Check sheet for the drawn part. Datum: minimum x, y, z corner. Units: mm. A direction names the side the tool comes from. Coordinates: 2 decimals unless noted, no trailing zeros. Write each loop counter-clockwise with the first axis right and the second up, starting at its lowest first coordinate (ties: lowest second). Pieces come first, ordered by that corner, then holes. Notation, with made-up numbers: (57, 6) -> (78, 6) arc R14 cw to (78, 31) -> close; hole circle Ø9 at (-12.75, -29). An arc over 180 degrees is marked (long way). Write item = value, one per line. Start each with the question number.
(1) Section check B-B (y = 9). Record the cut outline in (x, z), plus the area to 3 significant figures.
(2) Section check D-D (y = 19). Record the cut outline in (x, z), plus the area to 3 significant figures.
(3) Section check C-C (x = 32.5). Record the cut outline in (y, z), plus the area to 3 significant figures.
(4) Material ranges on probe 1 along Y at (x, z) = (32.5, 1.65); probe 2 along Y at (x, z) = (10, 0.8); probe 3 along Y at (x, z) = (20.5, 6), recorded low to high. Write a range as [from, to].
(5) Set-up check for the marked faces 1, 2 and 3: record each of +Z, -Z, +X, -X, +Y, -Y from which the full face is reachable in a straight line by a thin tool's end or side.
(6) Section check A-A (y = 42.5). Record the cut outline in (x, z), plus the area to 3 significant figures.
(7) Gauge pin test, flat ends, axial feed: pin 1 Ø3 at (y, z) = (35.5, 3) entering from -X; pin 2 Ø10 at (y, z) = (10, 4) entering from +X; pin 3 Ø3 at (x, y) = (23.5, 14) entering from +Z. Record the tip position at first contact, or that the pin passes through.
(8) Mould release check, pull along Y, two halves, no side actions. Record for the marked faces 4, 5 and 6: released by +Y, released by -Y, zero draft, split by the parting line, or undercut.
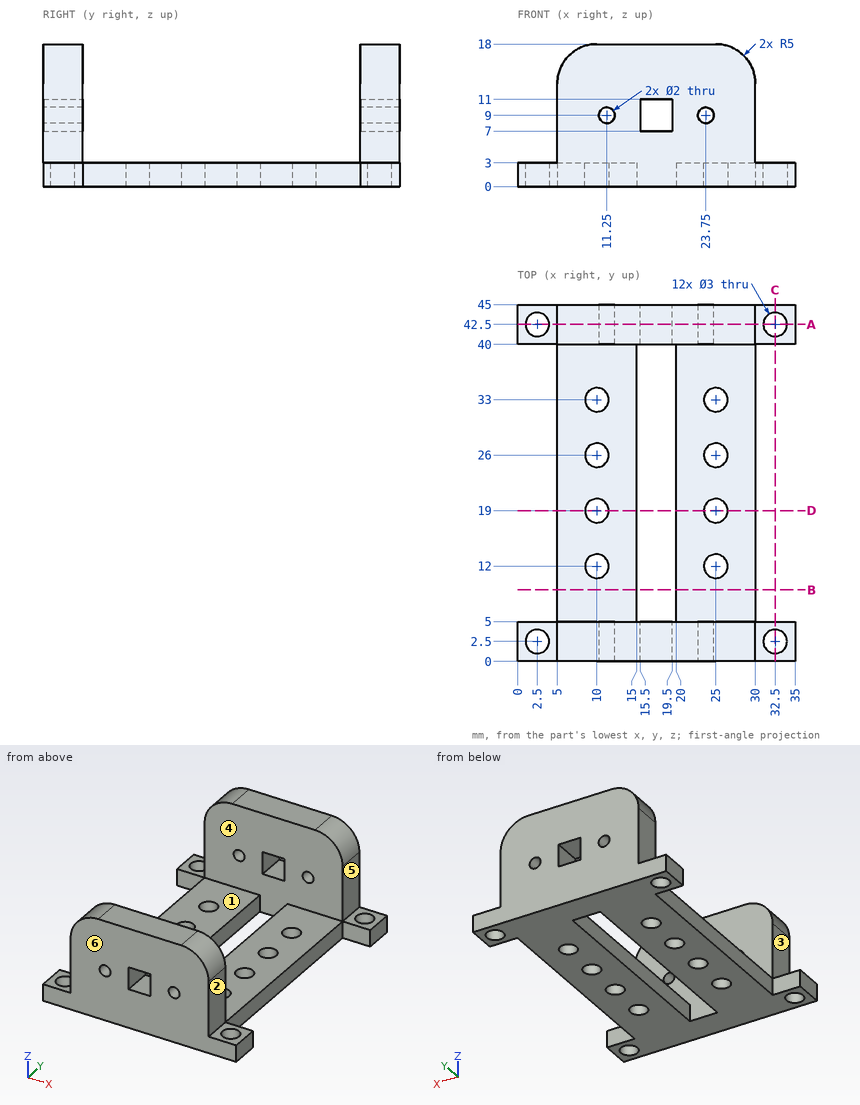
Response:
q1.outline = (5, 0) -> (15, 0) -> (15, 3) -> (5, 3) -> close; (20, 0) -> (30, 0) -> (30, 3) -> (20, 3) -> close
q1.area = 60.0 mm2
q2.outline = (5, 0) -> (8.5, 0) -> (8.5, 3) -> (5, 3) -> close; (11.5, 0) -> (15, 0) -> (15, 3) -> (11.5, 3) -> close; (20, 0) -> (23.5, 0) -> (23.5, 3) -> (20, 3) -> close; (26.5, 0) -> (30, 0) -> (30, 3) -> (26.5, 3) -> close
q2.area = 42.0 mm2
q3.outline = (0, 0) -> (1, 0) -> (1, 3) -> (0, 3) -> close; (4, 0) -> (5, 0) -> (5, 3) -> (4, 3) -> close; (40, 0) -> (41, 0) -> (41, 3) -> (40, 3) -> close; (44, 0) -> (45, 0) -> (45, 3) -> (44, 3) -> close
q3.area = 12.0 mm2
q4.probe_1 = [0, 1], [4, 5], [40, 41], [44, 45]
q4.probe_2 = [0, 10.5], [13.5, 17.5], [20.5, 24.5], [27.5, 31.5], [34.5, 45]
q4.probe_3 = [0, 5], [40, 45]
q5.face_1 = +Z, +X, -X
q5.face_2 = +Z, +X, +Y, -Y
q5.face_3 = +Z, -X, +Y, -Y
q6.outline = (0, 0) -> (1, 0) -> (1, 3) -> (0, 3) -> close; (4, 0) -> (31, 0) -> (31, 3) -> (30, 3) -> (30, 13) arc R5 ccw to (25, 18) -> (10, 18) arc R5 ccw to (5, 13) -> (5, 3) -> (4, 3) -> close; (34, 0) -> (35, 0) -> (35, 3) -> (34, 3) -> close; hole circle Ø2 at (11.25, 9); hole (15.5, 7) -> (19.5, 7) -> (19.5, 11) -> (15.5, 11) -> close; hole circle Ø2 at (23.75, 9)
q6.area = 429 mm2
q7.pin_1 = 5
q7.pin_2 = 30
q7.pin_3 = 3
q8.face_4 = undercut
q8.face_5 = zero draft
q8.face_6 = released by -Y
